Read the model definition and answer for the solid it produces. Units are mm, in the model's axes. A direction names the side the tool comes from. Give positions to 0.01 mm unless a question says otherwise; leave off trailing zeros. Order: outer loops, then holes, each group sorted by start corner. A loop starts at its lowest first (then second) coordinate and runs counter-clockwise, first axis right, second up. Notation, with made-up numbers: (79, 5.25) -> (87, 5.25) arc R25 cw to (87, 33.25) -> close; hole circle Ø6 at (88.25, -10). An arc over 180 degrees is marked (long way). Use one line per item in the form item = value.
```python
from build123d import *

# Parameters (mm, degrees)
SKETCH1_W           = 10.5
SKETCH1_H           = 5
BOSS_EXTRUDE1_DEPTH = 18
SKETCH2_W           = 10.5
SKETCH2_H           = 5
BOSS_EXTRUDE2_DEPTH = 7.3
SKETCH3_W           = 10.5
SKETCH3_H           = 1.95
CUT_EXTRUDE1_DEPTH  = 7.3
SKETCH4_W           = 10.5
SKETCH4_H           = 2.5
CUT_EXTRUDE2_DEPTH  = 26.3
SKETCH5_R           = 1.5
CUT_EXTRUDE3_DEPTH  = 26.3
SKETCH6_W           = 1.13
SKETCH6_H           = 3.05
CUT_EXTRUDE4_DEPTH  = 26.3
SKETCH10_W          = 10.5
SKETCH10_H          = 3.05
BOSS_EXTRUDE3_DEPTH = 5.5
SKETCH11_R          = 0.75
CUT_EXTRUDE6_DEPTH  = 12.5
SKETCH12_W          = 2
SKETCH12_H          = 1
CUT_EXTRUDE7_DEPTH  = 12.5


with BuildPart() as part:
    # Sketch1 → Boss-Extrude1 (new body)
    with BuildSketch(Plane(origin=(0, 0, 0), x_dir=(1, 0, 0), z_dir=(0, 1, 0))):
        Rectangle(SKETCH1_W, SKETCH1_H)
    extrude(amount=BOSS_EXTRUDE1_DEPTH)

    # Sketch2 → Boss-Extrude2 (add)
    with BuildSketch(Plane.XY.offset(2.5)):
        with Locations((0, 15.5)):
            Rectangle(SKETCH2_W, SKETCH2_H)
    extrude(amount=BOSS_EXTRUDE2_DEPTH)

    # Sketch3 → Cut-Extrude1 (cut)
    with BuildSketch(Plane.XY.offset(9.8)):
        with Locations((0, 13.975)):
            Rectangle(SKETCH3_W, SKETCH3_H)
    extrude(amount=-CUT_EXTRUDE1_DEPTH, mode=Mode.SUBTRACT)

    # Sketch4 → Cut-Extrude2 (cut)
    with BuildSketch(Plane(origin=(0, 0, 0), x_dir=(-1, 0, 0), z_dir=(0, -1, 0))):
        with Locations((0, 1.25)):
            Rectangle(SKETCH4_W, SKETCH4_H)
    extrude(amount=-CUT_EXTRUDE2_DEPTH, mode=Mode.SUBTRACT)

    # Sketch5 → Cut-Extrude3 (cut)
    with BuildSketch(Plane(origin=(0, 0, 0), x_dir=(-1, 0, 0), z_dir=(0, 0, -1))):
        with Locations((0, 4.5)):
            Circle(SKETCH5_R)
    extrude(amount=-CUT_EXTRUDE3_DEPTH, mode=Mode.SUBTRACT)

    # Sketch6 → Cut-Extrude4 (cut)
    with BuildSketch(Plane.ZY.offset(5.25)):
        with Locations((9.235, 16.475)):
            Rectangle(SKETCH6_W, SKETCH6_H)
    extrude(amount=-CUT_EXTRUDE4_DEPTH, mode=Mode.SUBTRACT)

    # Sketch10 → Boss-Extrude3 (add)
    with BuildSketch(Plane.XY.offset(8.67)):
        with Locations((0, 16.475)):
            Rectangle(SKETCH10_W, SKETCH10_H)
    extrude(amount=BOSS_EXTRUDE3_DEPTH)

    # Sketch11 → Cut-Extrude6 (cut)
    with BuildSketch(Plane.ZY.offset(5.25)):
        with Locations((11.3, 16.475)):
            Circle(SKETCH11_R)
    extrude(amount=-CUT_EXTRUDE6_DEPTH, mode=Mode.SUBTRACT)

    # Sketch12 → Cut-Extrude7 (cut)
    with BuildSketch(Plane.ZY.offset(5.25)):
        with Locations((13.17, 15.45)):
            Rectangle(SKETCH12_W, SKETCH12_H)
    extrude(amount=-CUT_EXTRUDE7_DEPTH, mode=Mode.SUBTRACT)


solid = part.part
```
Item 1: The part is cut by section A-A on z = 11.3. Give the vertices of the cut face in (x, y) (3 decimals).
Checks:
outline = (-5.25, 14.95) -> (5.25, 14.95) -> (5.25, 15.725) -> (-5.25, 15.725) -> close; (-5.25, 17.225) -> (5.25, 17.225) -> (5.25, 18) -> (-5.25, 18) -> close
Item 2: Determine the mould class of faces 3 (the flat face through (0, 7, 2.5)), 4 (the cylindrical face through (1.5, 4.57, 1.23)), 5 (the flat face through (0, 0, 1)) for opening direction Y: +Y half, -Y half, draft (parallel to the pull), parting line (faces both ways), or undercut.
Checks:
face_3 = draft
face_4 = undercut
face_5 = -Y half
Item 3: The part is cut by section B-B on y = 4.5. Give the vertices of the cut face in (x, z), and give its area (4 significant figures).
Checks:
outline = (-5.25, 0) -> (-1.5, 0) -> (-1.5, 2.5) -> (-5.25, 2.5) -> close; (1.5, 0) -> (5.25, 0) -> (5.25, 2.5) -> (1.5, 2.5) -> close
area = 18.75 mm²
Item 4: The part is cut by section D-D on x = -3. Give the vertices of the cut face in (y, z) (3 decimals).
Checks:
outline = (0, 0) -> (18, 0) -> (18, 14.17) -> (15.95, 14.17) -> (15.95, 12.17) -> (14.95, 12.17) -> (14.95, 2.5) -> (0, 2.5) -> close; hole circle Ø1.5 at (16.475, 11.3)
Item 5: Given pin 1 Ø2 at (x, z) = (-4, 12) entering from -Y; pin 2 Ø1 at (x, z) = (1.5, 13.5) entering from -Y; pin 3 Ø5 at (x, y) = (-1.5, 10.5) entering from +Z; pin 4 Ø2.5 at (x, y) = (0, 4.5) entering from +Z, each flat-ended and moving along its own axis, determine where each tip first touches the part or whether it passes through.
Checks:
pin_1 = 14.95
pin_2 = 15.95
pin_3 = 2.5
pin_4 = through
Item 6: The part is cut by section C-C on x = -0.25. Give the vertices of the cut face in (y, z) (3 decimals), and give its area (3 significant figures).
Checks:
outline = (0, 0) -> (3.021, 0) -> (3.021, 2.5) -> (0, 2.5) -> close; (5.979, 0) -> (18, 0) -> (18, 14.17) -> (15.95, 14.17) -> (15.95, 12.17) -> (14.95, 12.17) -> (14.95, 2.5) -> (5.979, 2.5) -> close; hole circle Ø1.5 at (16.475, 11.3)
area = 69.4 mm²
Item 7: Which of the six approach directions +Z, -Z, +X, -X, +Y, -Y give full straight-line access (tool end or side, diameter ignored) to faces 1 (the flat face through (0, 17, 14.17)), 2 (the flat face through (0, 14.95, 7))?
Checks:
face_1 = +Z, +X, -X, +Y, -Y
face_2 = +Z, +X, -X, -Y
Item 8: Straight lines are drawn through the part: L1, parallel to Y at x = 0, z = 0.85; L2, parallel to Y at x = -1.5, z = 11.25; L3, parallel to Y at x = 4, z = 7.75. For each, find the intervals that lie inside material, in ascending order. Write a range as from..to.
Checks:
L1 = 0..3, 6..18
L2 = 14.95..15.73, 17.22..18
L3 = 14.95..18
